from build123d import *

# Parameters (mm, degrees)
F0_W      = 144.6334645152
F0_H      = 5.0355943386
F1_DEPTH  = 25.4
F3_DEPTH  = 2.54
F5_DEPTH  = 2.54
F6_W      = 102.6701740921
F6_H      = 25.2759195864
F7_DEPTH  = 0.254
F8_W      = 3.4340582788
F8_H      = 30.7748552877
F9_DEPTH  = 2.54
F10_W     = 3.6297179759
F10_H     = 32.1495756507
F11_DEPTH = 2.54
F12_W     = 3.6330670118
F12_H     = 30.970800959
F13_DEPTH = 2.54
F14_W     = 3.4567825496
F14_H     = 30.4196920479
F15_DEPTH = 2.54
F17_DEPTH = 2.54
F19_DEPTH = 2.54
F20_W     = 5.5748282466
F20_H     = 6.0991924256
F21_DEPTH = 33.02
F22_W     = 3.5782083869
F22_H     = 4.1668945923
F23_DEPTH = 33.02
F24_W     = 2.8318321891
F24_H     = 5.08
F25_DEPTH = 33.02
F26_W     = 167.146153748
F26_H     = 1.6835723072
F27_DEPTH = 25.4
F28_W     = 29.1326753795
F28_H     = 25.4
F29_DEPTH = 10.16
F30_W     = 29.6150818467
F30_H     = 25.4
F31_DEPTH = 10.16


with BuildPart() as f1:
    # F0 (on Front) → F1 (new body)
    with BuildSketch(Plane.XZ):
        with Locations((0.2797581255, -0.1398775494)):
            Rectangle(F0_W, F0_H)
    extrude(amount=F1_DEPTH)

    # F2 (on Front) → F3 (join)
    with BuildSketch(Plane.XZ):
        Polygon((-72.0369741321, 2.6576747186), (-72.0369741321, 0), (-69.2392249852, 0), (-69.2392249852, 2.6093864363), (-50.4433400929, 30.9355836362), (48.9940978587, 30.9355836362), (69.989785552, 2.1328825969), (69.989785552, 0), (72.3275691271, 0), (72.3275691271, 2.345408313), (50.4958182573, 32.5914844871), (-52.1743558347, 32.5914844871), align=None)
    extrude(amount=F3_DEPTH)

    # F4 (on face) → F5 (join)
    with BuildSketch(Plane.XZ.offset(25.4)):
        Polygon((-72.0369741321, 2.3779196199), (-72.0369741321, -0.1398775494), (-68.5875401776, 0), (-68.5875401776, 2.3779196199), (-49.9622374773, 31.0818161815), (49.0318536758, 31.0818161815), (70.0765177608, 2.3779196199), (70.0765177608, 0), (72.5964903831, 0), (72.5964903831, 2.3779196199), (50.2103567123, 32.7653884888), (-52.319239825, 32.7653884888), align=None)
    extrude(amount=-F5_DEPTH)

    # F6 (on face) → F7 (join)
    with BuildSketch(Plane.XY.offset(32.5914844871)):
        with Locations((-0.8392687887, -12.6379597932)):
            Rectangle(F6_W, F6_H)
    extrude(amount=F7_DEPTH)

    # F8 (on face) → F9 (join)
    with BuildSketch(Plane.XZ.offset(25.4)):
        with Locations((-48.2452083379, 16.5978105506)):
            Rectangle(F8_W, F8_H)
    extrude(amount=-F9_DEPTH)

    # F10 (on face) → F11 (join)
    with BuildSketch(Plane.XZ.offset(25.4)):
        with Locations((47.2169946879, 16.0747878253)):
            Rectangle(F10_W, F10_H)
    extrude(amount=-F11_DEPTH)

    # F12 (on face) → F13 (join)
    with BuildSketch(Plane(origin=(0, 0, 0), x_dir=(-1, 0, 0), z_dir=(0, 1, 0))):
        with Locations((-47.1775643528, 16.3971947914)):
            Rectangle(F12_W, F12_H)
    extrude(amount=-F13_DEPTH)

    # F14 (on face) → F15 (join)
    with BuildSketch(Plane(origin=(0, 0, 0), x_dir=(-1, 0, 0), z_dir=(0, 1, 0))):
        with Locations((48.3132656664, 16.6731329518)):
            Rectangle(F14_W, F14_H)
    extrude(amount=-F15_DEPTH)

    # F16 (on face) → F17 (join)
    with BuildSketch(Plane(origin=(0, 0, 0), x_dir=(-1, 0, 0), z_dir=(0, 1, 0))):
        Polygon((-45.3610308468, 31.9995991886), (-47.1585355699, 30.9355836362), (0, 0), (48.751424998, 30.9355836362), (47.5394830392, 32.8454844871), (0, 2.678947742), align=None)
    extrude(amount=-F17_DEPTH)

    # F18 (on face) → F19 (join)
    with BuildSketch(Plane.XZ.offset(25.4)):
        Polygon((-46.5281791985, 32.2389304638), (-48.4291017056, 31.0818161815), (0, 0), (47.5102737546, 31.0818161815), (45.4021357, 32.7653884888), (0, 3.0627426281), align=None)
    extrude(amount=-F19_DEPTH)

    # F20 (on face) → F21 (join)
    with BuildSketch(Plane(origin=(0, 0, 32.5914844871), x_dir=(1, 0, 0), z_dir=(0, 0, -1))):
        with Locations((-0.5173498066, 12.4324662611)):
            Rectangle(F20_W, F20_H)
    extrude(amount=F21_DEPTH)

    # F22 (on face) → F23 (join)
    with BuildSketch(Plane(origin=(0, 0, 32.5914844871), x_dir=(1, 0, 0), z_dir=(0, 0, -1))):
        with Locations((-48.0833910406, 12.3338256963)):
            Rectangle(F22_W, F22_H)
    extrude(amount=F23_DEPTH)

    # F24 (on face) → F25 (join)
    with BuildSketch(Plane(origin=(0, 0, 32.5914844871), x_dir=(1, 0, 0), z_dir=(0, 0, -1))):
        with Locations((47.2405347973, 11.4395930432)):
            Rectangle(F24_W, F24_H)
    extrude(amount=F25_DEPTH)

    # F26 (on face) → F27 (join)
    with BuildSketch(Plane.XZ.offset(25.4)):
        with Locations((0.1240931451, 31.9236023352)):
            Rectangle(F26_W, F26_H)
    extrude(amount=-F27_DEPTH)

    # F28 (on face) → F29 (join)
    with BuildSketch(Plane(origin=(0, 0, -2.6576747186), x_dir=(1, 0, 0), z_dir=(0, 0, -1))):
        with Locations((-57.4706364423, 12.7)):
            Rectangle(F28_W, F28_H)
    extrude(amount=F29_DEPTH)

    # F30 (on face) → F31 (join)
    with BuildSketch(Plane(origin=(0, 0, -2.6576747186), x_dir=(1, 0, 0), z_dir=(0, 0, -1))):
        with Locations((57.7889494598, 12.7)):
            Rectangle(F30_W, F30_H)
    extrude(amount=F31_DEPTH)


solid = f1.part
Here's how the part is built. I have some questions about the finished solid (model axes, mm). A direction names the side the tool comes from. Coordinates: 2 decimals unless noted, no trailing zeros. Order: outer loops, then holes, each group sorted by start corner. A loop starts at its lowest first (then second) coordinate and runs counter-clockwise, first axis right, second up. Notation, with made-up numbers: (-12, 11) - (0, 11) arc R34 cw to (0, 44) - close; hole circle Ø3 at (0.5, 47.5). An arc over 180 degrees is marked (long way). Use CSV: the item, a comma, the result in double quotes. Start each with the question number.
1. Suppose I cut it at D-D on x = -16.5. List the corners of the cut face in (y, z) for me, then the cut area to 3 significant figures.
2. For faces 1 (the face through (45.825, -11, 17)), 2 (the face through (-59.405, -24.148, 16.529)), 3 (the face through (-48, -10.25, 17)), 4 (the face through (47, -8.9, 17)), which set-ups out of +Z, -Z, +X, -X, +Y, -Y let a thin tool reach every point of the face, with its end or its side?
3. If we mould it in two halves opening along Y, with no side actions, what happens to faces 5 (the face through (-6, -25.4, 5)), 6 (the face through (24.23, -24.15, 15.85)), 7 (the face through (48.656, -11, 17))? For each: +Y half, -Y half, draft (parallel to the pull), parting line (faces both ways), or undercut.
4. Please list where these lines run through material, in increasing order: line 1 (X direction, y = -11.75, z = 18); line 2 (Z direction, x = -61, y = -5.5); line 3 (Z direction, x = -6, y = -8.5). Write a range as from..to.
5. I'm going to push flat-ended pins straight in: pin 1 (12.5 mm diameter, centred on x = 15.5, y = -11, fed in from -Z); pin 2 (2 mm diameter, centred on y = -9, z = 3.5, fed in from +X); pin 3 (2 mm diameter, centred on y = -21, z = 27.5, fed in from +X); pin 4 (3 mm diameter, centred on y = -23.5, z = 17, fed in from -X). Where does each tip first touch, or does it pass through?
6. Suppose I cut it at C-C on x = 30. List the corners of the cut face in (y, z) for me.
7. Suppose I cut it at B-B on z = -9. List the corners of the cut face in (x, y) for me.
8. Suppose I cut it at A-A on y = -5. List the corners of the cut face in (x, z) for me.
Output:
1,outline,"(-25.4, -2.66) - (0, -2.66) - (0, 2.38) - (-25.4, 2.38) - close; (-25.4, 10.59) - (-22.86, 10.59) - (-22.86, 13.41) - (-25.4, 13.41) - close; (-25.4, 31.08) - (-2.54, 31.08) - (-2.54, 30.94) - (0, 30.94) - (0, 32.85) - (-25.28, 32.85) - (-25.28, 32.77) - (-25.4, 32.77) - close; (-2.54, 10.47) - (0, 10.47) - (0, 13.15) - (-2.54, 13.15) - close"
1,area,"187 mm2"
2,face 1,"none"
2,face 2,"+Y, -Y"
2,face 3,"-X"
2,face 4,"+X, -X"
3,face 5,"-Y half"
3,face 6,"draft"
3,face 7,"undercut"
4,line 1,"x = -49.87..-46.29, -3.3..2.27, 45.82..48.66"
4,line 2,"z = -12.82..2.38, 31.08..32.77"
4,line 3,"z = -2.66..2.38, 31.08..32.85"
5,pin 1,"stops at z = -2.66"
5,pin 2,"stops at x = 48.66"
5,pin 3,"passes through"
5,pin 4,"stops at x = -63.52"
6,outline,"(-25.4, -2.66) - (0, -2.66) - (0, 2.38) - (-25.4, 2.38) - close; (-25.4, 19.63) - (-22.86, 19.63) - (-22.86, 22.69) - (-25.4, 22.69) - close; (-25.4, 31.08) - (-2.54, 31.08) - (-2.54, 30.94) - (0, 30.94) - (0, 32.85) - (-25.28, 32.85) - (-25.28, 32.77) - (-25.4, 32.77) - close; (-2.54, 19.68) - (0, 19.68) - (0, 22.07) - (-2.54, 22.07) - close"
7,outline,"(-72.04, -25.4) - (-42.9, -25.4) - (-42.9, 0) - (-72.04, 0) - close; (42.98, -25.4) - (72.6, -25.4) - (72.6, 0) - (42.98, 0) - close"
8,outline,"(-83.45, 31.08) - (83.7, 31.08) - (83.7, 32.77) - (50.5, 32.77) - (50.5, 32.85) - (-52.17, 32.85) - (-52.17, 32.77) - (-83.45, 32.77) - close; (-72.04, -12.82) - (-42.9, -12.82) - (-42.9, -2.66) - (42.98, -2.66) - (42.98, -12.82) - (72.6, -12.82) - (72.6, 2.38) - (-72.04, 2.38) - close"
